```python
from build123d import *

# Parameters (mm, degrees)
BOSS_EXTRUDE1_DEPTH = 6.4
CHAMFER3_SIZE       = 2
CUT_EXTRUDE1_DEPTH  = 0.85
CUT_EXTRUDE2_DEPTH  = 0.85


with BuildPart() as part:
    # Sketch1 → Boss-Extrude1 (new body)
    with BuildSketch(Plane(origin=(0, 0, 0), x_dir=(0, 0, -1), z_dir=(1, 0, 0))):
        with BuildLine():
            Line((0, 0.1), (0, 7.05))
            Line((0, 7.05), (-0.241393443, 8.15))
            Line((-0.241393443, 8.15), (-0.647131148, 8.15))
            Line((-0.647131148, 8.15), (-0.85, 7.05))
            Line((-0.85, 7.05), (-0.85, -0.1))
            ThreePointArc((-0.85, -0.1), (-0.630330086, -0.630330086), (-0.1, -0.85))
            Line((-0.1, -0.85), (5.15, -0.85))
            Line((5.15, -0.85), (5.15, 0))
            Line((5.15, 0), (0.1, 0))
            ThreePointArc((0.1, 0), (0.029289322, 0.029289322), (0, 0.1))
        make_face()
    extrude(amount=BOSS_EXTRUDE1_DEPTH)

    # Chamfer3
    chamfer3_edges = [part.edges().sort_by_distance(p)[0] for p in [
        (0, -0.425, -5.15),
        (6.4, -0.425, -5.15),
    ]]
    chamfer(chamfer3_edges, length=CHAMFER3_SIZE)

    # Sketch4 → Cut-Extrude1 (cut)
    with BuildSketch(Plane.XY.offset(0.85)):
        Polygon((0, 6.9), (1.25, 8.15), (0, 8.15), align=None)
        Polygon((5.15, 8.15), (6.4, 6.9), (6.4, 8.15), align=None)
    extrude(amount=-CUT_EXTRUDE1_DEPTH, mode=Mode.SUBTRACT)

    # Sketch5 → Cut-Extrude2 (cut)
    with BuildSketch(Plane.XY.offset(0.85)):
        with BuildLine():
            Line((2.730622244, 5.748829869), (2.026555611, 3.830729922))
            ThreePointArc((2.026555611, 3.830729922), (3.20000017, 2.15), (4.373444272, 3.830730241))
            Line((4.373444272, 3.830730241), (3.669633952, 5.748130298))
            ThreePointArc((3.669633952, 5.748130298), (3.200372504, 6.076537762), (2.730622244, 5.748829869))
        make_face()
    extrude(amount=-CUT_EXTRUDE2_DEPTH, mode=Mode.SUBTRACT)


solid = part.part
```
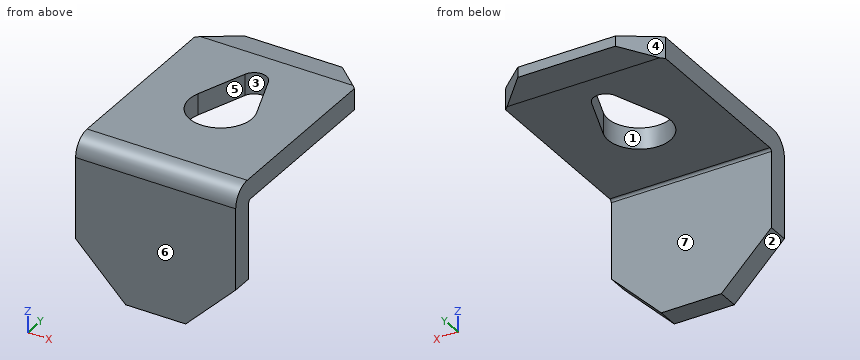
The listing builds one solid part. Answer for the finished solid, in the listing's coordinates (mm). Face numbers are marked on the shaded views. A direction names the side the tool comes from. Coordinates: 2 decimals unless noted, no trailing zeros. Write each loop counter-clockwise with the first axis right and the second up, starting at its lowest first coordinate (ties: lowest second). Pieces come first, ordered by that corner, then holes. Notation, with made-up numbers: (56, 35) - (78, 35) arc R23 cw to (78, 60) - close; hole circle Ø7 at (-30.5, 1). An arc over 180 degrees is marked (long way). Return JSON: item names as keys, results as strings. Group by question number.
Q1. Which of the six approach directions +Z, -Z, +X, -X, +Y, -Y give full straight-line access (tool end or side, diameter ignored) to the marked faces 5, 6 and 7?
Q2. Flat-ended cylindrical pins translate along their axes: pin 1 Ø3 at (x, y) = (4, 2.5) entering from -Z; pin 2 Ø2 at (x, z) = (3, -3) entering from +Y. Find the tip coordinate at first contact, or state that the pin passes through.
Q3. The part is cut by section B-B on y = 3.4. Write down the section's boundary in (x, z).
Q4. For a pull along Y with two mould halves and no side action, classify the marked faces 1, 2, 3 and 4 as +Y half, -Y half, draft (parallel to the pull), parting line (faces both ways), or undercut.
Q5. The part is cut by section D-D on y = 1. Write down the section's boundary in (x, z).
Q6. The part is cut by section A-A on x = 3.2. Write down the section's boundary in (y, z).
Q7. The part is cut by section C-C on z = -2.3. Write down the section's boundary in (x, y).
Q8. Find the intervals of material crossed by line 1 along X through (y, z) = (3.4, 0.2); line 2 along Y through (x, z) = (6, -0.1); line 3 along Z through (x, y) = (1.75, 2.5), in increasing order. Write a range as [from, to].
Evaluation:
{
 "1": {"face 5": "+Z, -Z", "face 6": "+Z, -Z, +X, -X, -Y", "face 7": "-Z, +X, -X, +Y"},
 "2": {"pin 1": "stops at z = 0", "pin 2": "stops at y = 0"},
 "3": {"outline": "(0, 0) - (1.95, 0) - (1.95, 0.85) - (0, 0.85) - close; (4.45, 0) - (6.4, 0) - (6.4, 0.85) - (4.45, 0.85) - close"},
 "4": {"face 1": "undercut", "face 2": "draft", "face 3": "undercut", "face 4": "+Y half"},
 "5": {"outline": "(0, 0) - (6.4, 0) - (6.4, 0.85) - (0, 0.85) - close"},
 "6": {"outline": "(-0.85, -5.15) - (0, -5.15) - (0, -0.1) arc R0.1 cw to (0.1, 0) - (2.15, 0) - (2.15, 0.85) - (-0.1, 0.85) arc R0.75 ccw to (-0.85, 0.1) - close; (6.08, 0) - (7.05, 0) - (8.15, 0.24) - (8.15, 0.65) - (7.05, 0.85) - (6.08, 0.85) - close"},
 "7": {"outline": "(0, -0.85) - (6.4, -0.85) - (6.4, 0) - (0, 0) - close"},
 "8": {"line 1": "x = [0, 1.95], [4.45, 6.4]", "line 2": "y = [-0.85, 0]", "line 3": "z = [0, 0.85]"}
}
